Verification items for this drawing (mm, ordinates from the low corner). Coordinates: 2 decimals unless noted, no trailing zeros. Order: outer loops, then holes, each group sorted by start corner. A loop starts at its lowest first (then second) coordinate and runs counter-clockwise, first axis right, second up. Notation, with made-up numbers: (2.5, -13) -> (11.5, -13) arc R20 ccw to (11.5, -6) -> close; hole circle Ø7 at (63, -10). An arc over 180 degrees is marked (long way). Write each question's results on one line, items separated by ' | '. Start each with the question number.
(1) Go/stop test with a flat-tipped pin: pin 1 (4 mm diameter, centred on x = 19.05, y = 19.05, fed in from -Z). Record where the tip stops, or that it passes through.
(2) Thickness scan on probe 1 along Y at (x, z) = (234.95, 1); probe 2 along X at (y, z) = (18, 1.45). Record the ranges inside material, lowest first. Write a range as [from, to].
(3) Cross-section at B-B on x = 234.95. Enter the section's corners in (y, z).
(4) Cross-section at A-A on y = 19.05. Enter the section's corners in (x, z).
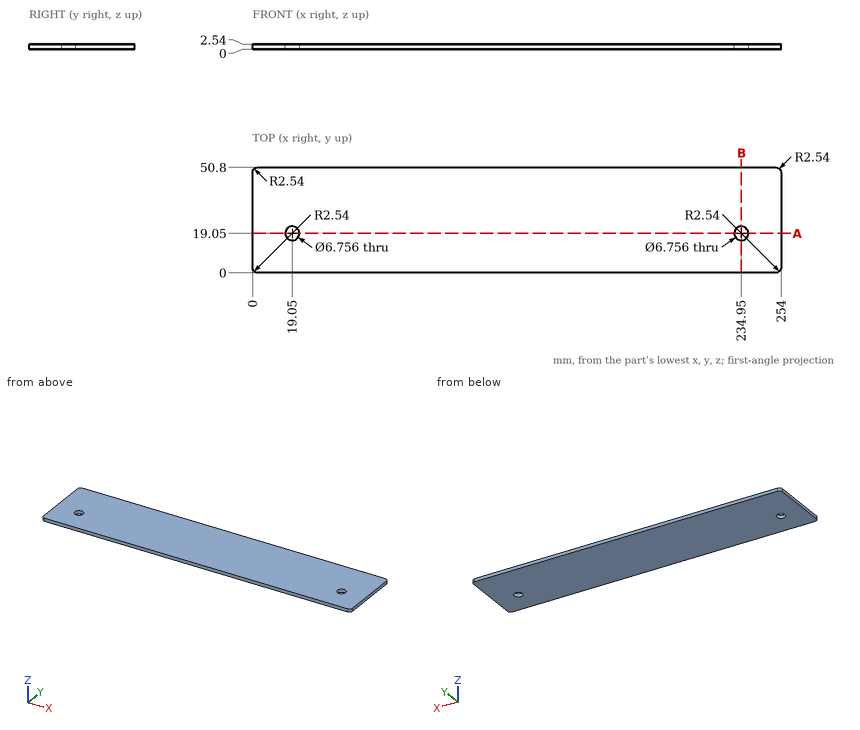
Results are:
1) pin 1: passes through
2) probe 1: y = [0, 15.67], [22.43, 50.8] | probe 2: x = [0, 15.84], [22.26, 231.74], [238.16, 254]
3) outline: (0, 0) -> (15.67, 0) -> (15.67, 2.54) -> (0, 2.54) -> close; (22.43, 0) -> (50.8, 0) -> (50.8, 2.54) -> (22.43, 2.54) -> close
4) outline: (0, 0) -> (15.67, 0) -> (15.67, 2.54) -> (0, 2.54) -> close; (22.43, 0) -> (231.57, 0) -> (231.57, 2.54) -> (22.43, 2.54) -> close; (238.33, 0) -> (254, 0) -> (254, 2.54) -> (238.33, 2.54) -> close
